```python
from build123d import *

# Parameters (mm, degrees)
F1_DEPTH = 3


with BuildPart() as f1:
    # F0 (on Top) → F1 (new body)
    with BuildSketch(Plane.XY):
        with BuildLine():
            ThreePointArc((-29.98936, 27.868279), (-36.55688, 30.159424), (-42.43597, 26.442172))
            ThreePointArc((-42.43597, 26.442172), (-50, 0), (-42.43597, -26.442172))
            ThreePointArc((-42.43597, -26.442172), (-36.55688, -30.159424), (-29.98936, -27.868279))
            Line((-29.98936, -27.868279), (-22.273744, -20.152663))
            Line((-22.273744, -20.152663), (-20.152663, -22.273744))
            Line((-20.152663, -22.273744), (-27.868279, -29.98936))
            ThreePointArc((-27.868279, -29.98936), (-30.159424, -36.55688), (-26.442172, -42.43597))
            ThreePointArc((-26.442172, -42.43597), (0, -50), (26.442172, -42.43597))
            ThreePointArc((26.442172, -42.43597), (30.159424, -36.55688), (27.868279, -29.98936))
            Line((27.868279, -29.98936), (20.152663, -22.273744))
            Line((20.152663, -22.273744), (22.273744, -20.152663))
            Line((22.273744, -20.152663), (29.98936, -27.868279))
            ThreePointArc((29.98936, -27.868279), (36.55688, -30.159424), (42.43597, -26.442172))
            ThreePointArc((42.43597, -26.442172), (50, 0), (42.43597, 26.442172))
            ThreePointArc((42.43597, 26.442172), (36.55688, 30.159424), (29.98936, 27.868279))
            Line((29.98936, 27.868279), (22.273744, 20.152663))
            Line((22.273744, 20.152663), (20.152663, 22.273744))
            Line((20.152663, 22.273744), (27.868279, 29.98936))
            ThreePointArc((27.868279, 29.98936), (30.159424, 36.55688), (26.442172, 42.43597))
            ThreePointArc((26.442172, 42.43597), (0, 50), (-26.442172, 42.43597))
            ThreePointArc((-26.442172, 42.43597), (-30.159424, 36.55688), (-27.868279, 29.98936))
            Line((-27.868279, 29.98936), (-20.189875, 22.310956))
            Line((-20.189875, 22.310956), (-22.110491, 19.989409))
            Line((-22.110491, 19.989409), (-29.98936, 27.868279))
        make_face()
        Polygon((-1.5, 30), (1.5, 30), (1.5, 3.621082), (1.5, 1.5), (3.621082, 1.5), (30, 1.5), (30, -1.5), (3.621082, -1.5), (1.5, -1.5), (1.5, -3.621082), (1.5, -30), (-1.5, -30), (-1.5, -3.621082), (-1.5, -1.5), (-3.621082, -1.5), (-30, -1.5), (-30, 1.5), (-3.621082, 1.5), (-1.5, 1.5), (-1.5, 3.621082), align=None, mode=Mode.SUBTRACT)
    extrude(amount=F1_DEPTH)


solid = f1.part
```
For this review, take the finished solid that the model builds, in its own axes (mm). A direction names the side the tool comes from. Give positions to 0.01 mm unless a question says otherwise; leave off trailing zeros. Order: outer loops, then holes, each group sorted by start corner. A loop starts at its lowest first (then second) coordinate and runs counter-clockwise, first axis right, second up.
1) Wall thickness on line 1 (X direction, y = -26, z = 2.25); line 2 (X direction, y = -21.5, z = 1.45); line 3 (Y direction, x = 21, z = 1.2): over which ranges is each line inside the solid? List them lowest first.
2) The part is to be moulded in two halves that separate along Y. For faces 1 (the face through (0, 30, 1)), 2 (the face through (10, -10, 3)), 3 (the face through (50, 0, 1)), say which applies: released by +Y, released by -Y, zero draft, split by the parting line, or undercut.
3) Insertion check: pin 1 (1 mm diameter, centred on y = 6, z = 1, fed in from +X); pin 2 (1 mm diameter, centred on x = 20, z = 2, fed in from -Y); pin 3 (0.9 mm diameter, centred on y = 19.5, z = 2, fed in from -X). Each pin has a flat end and moves straight along its axis. Give the tip position at first contact, or say it passes through.
4) For faces 4 (the face through (-23.96, -26.08, 1.48)), 5 (the face through (-50, 0, 1)), list the 3-axis set-ups (+Z, -Z, +X, -X, +Y, -Y) from which the entire face can be reached by the end or side of a thin tool; tool diameter is ignored.
5) Take a section at C-C (y = 44). Give the boundary of the cut face in (x, z).
6) Take a section at A-A (y = -9). Give the boundary of the cut face in (x, z), then the cut area to 3 significant figures.
7) Take a section at B-B (x = 35.5). Give the boundary of the cut face in (y, z), then the cut area to 3 significant figures.
Derived:
1. line 1: x = -42.71 to -28.12, -23.88 to -1.5, 1.5 to 23.88, 28.12 to 42.71
1. line 2: x = -45.14 to -23.62, -20.93 to -1.5, 1.5 to 20.93, 23.62 to 45.14
1. line 3: y = -45.38 to -23.12, -21.43 to -1.5, 1.5 to 21.43, 23.12 to 45.38
2. face 1: undercut
2. face 2: zero draft
2. face 3: split by the parting line
3. pin 1: stops at x = 49.7
3. pin 2: stops at y = -46.04
3. pin 3: stops at x = -46.23
4. face 4: +Z, -Z
4. face 5: +Z, -Z, -X
5. outline: (-23.75, 0) - (23.75, 0) - (23.75, 3) - (-23.75, 3) - close
6. outline: (-49.18, 0) - (-1.5, 0) - (-1.5, 3) - (-49.18, 3) - close; (1.5, 0) - (49.18, 0) - (49.18, 3) - (1.5, 3) - close
6. area: 286 mm2
7. outline: (-30.21, 0) - (30.21, 0) - (30.21, 3) - (-30.21, 3) - close
7. area: 181 mm2
